Part model, mm, in its own coordinate system. A direction names the side the tool comes from. Give positions to 0.01 mm unless a question says otherwise; leave off trailing zeros. Write each loop counter-clockwise with the first axis right and the second up, starting at its lowest first coordinate (ties: lowest second). Pieces come first, ordered by that corner, then holes. Notation, with made-up numbers: (72, 87.25) - (109, 87.25) arc R29 cw to (109, 118.25) - close; hole circle Ø6 at (5, -9). An arc over 180 degrees is marked (long way). Answer in a Markdown table with one row per item. Add a question column.
1. Band-saw the part on C-C on z = 0.25. Write the cut outline in (x, y), plus the area to 3 significant figures.
2. Drop flat-ended pins along their axis: pin 1 Ø0.6 at (x, z) = (-1.5, -0.5) entering from -Y; pin 2 Ø1.7 at (x, z) = (0.5, 3) entering from -Y; pin 3 Ø1 at (x, z) = (4.5, 2.5) entering from -Y. Give the stop position or say it passes through.
3. Which spindle directions (+Z, -Z, +X, -X, +Y, -Y) get a long thin tool onto all of the face, cutting with end or side? Do faces 4 (the flat face through (-9.88, -1.16, 2.75)), 5 (the cylindrical face through (6.976, 2.754, 0.128)), 6 (the flat face through (-1, -10, -1.5)). Say none if no direction does.
4. Probe line 1 along X through (y, z) = (0, 2.75); line 2 along Z through (x, y) = (6.5, -4.25); line 3 along X through (y, z) = (4.5, -6). List the from-to ranges inside material, lowest first.
5. Band-saw the part on B-B on y = -8.5. Write the cut outline in (x, z), plus the area to 3 significant figures.
6. Pull direction Y, two halves, no side cores. Call faces 1 (the cylindrical face through (-0.857, -9.467, -0.021)), 2 (the cylindrical face through (7.614, -2.612, -1.705)), 3 (the flat face through (-1, -10, 1.5)): released by +Y, released by -Y, zero draft, split by the parting line, or undercut.
```python
from build123d import *

# Parameters (mm, degrees)
RESSALTO_EXTRUS_O1_DEPTH  = 10
CORTE_EXTRUS_O8_OUTLINE_W = 20
CORTE_EXTRUS_O8_OUTLINE_H = 20
CORTE_EXTRUS_O8_DEPTH     = 8.5
RESSALTO_EXTRUS_O2_START  = 1
RESSALTO_EXTRUS_O2_DEPTH  = 1
VARREDURA3_START          = -1.500007282
VARREDURA3_DEPTH          = 3
CORTE_EXTRUS_O9_DEPTH     = 15.5
FILETE1_R                 = 5


# Read off the part's stored shape, not the designer's step: Corte-extrusão8, Varredura3
with BuildPart() as part:
    # Esboço1 → Ressalto-extrusão1 (new, symmetric)
    with BuildSketch(Plane.XY):
        with BuildLine():
            Line((0, 8.5), (0, 7))
            Line((0, 7), (2.692582404, 7))
            ThreePointArc((2.692582404, 7), (7.373940602, -1.369306394), (0, -7.5))
            Line((0, -7.5), (0, -8.5))
            ThreePointArc((0, -8.5), (8.5, 0), (0, 8.5))
        make_face()
    extrude(amount=RESSALTO_EXTRUS_O1_DEPTH, both=True)

    # Corte-extrusão8 outline → Corte-extrusão8 (cut)
    with BuildSketch(Plane(origin=(0, 0, 0), x_dir=(0, 0, -1), z_dir=(1, 0, 0))):
        Rectangle(CORTE_EXTRUS_O8_OUTLINE_W, CORTE_EXTRUS_O8_OUTLINE_H)
        with BuildLine():
            add(Edge.make_bspline(
                [(9.000007282, 4.914510614), (9.447062759, 5.785868524), (9.685629081, 6.469892836)],
                knots=[0, 0, 0, 0.163868034, 0.163868034, 0.163868034], degree=2))
            add(Edge.make_bspline(
                [(3.935539792, -0.04688611), (4.779617707, 0.456269007), (6.467773537, 1.786323577), (8.155929367, 3.763866822), (9.000007282, 4.914510614)],
                knots=[0.718640695, 0.718640695, 0.718640695, 0.718640695, 0.859320348, 1, 1, 1, 1], degree=3))
            ThreePointArc((3.935539792, -0.04688611), (3.567999305, -0.305127766), (3.243137148, -0.615352428))
            Line((3.243137148, -0.615352428), (2.271512773, -1.693435261))
            ThreePointArc((2.271512773, -1.693435261), (1.699517724, -2.626111152), (1.500007282, -3.701870529))
            Line((1.500007282, -3.701870529), (-1.499992718, -3.701870529))
            ThreePointArc((-1.499992718, -3.701870529), (-1.69950316, -2.626111152), (-2.271498209, -1.693435261))
            Line((-2.271498209, -1.693435261), (-3.243122584, -0.615352428))
            ThreePointArc((-3.243122584, -0.615352428), (-3.567984742, -0.305127766), (-3.935525229, -0.04688611))
            add(Edge.make_bspline(
                [(-8.999992718, 4.914510614), (-8.155914803, 3.763866822), (-6.467758973, 1.786323577), (-4.779603143, 0.456269007), (-3.935525229, -0.04688611)],
                knots=[0, 0, 0, 0, 0.140679652, 0.281359305, 0.281359305, 0.281359305, 0.281359305], degree=3))
            add(Edge.make_bspline(
                [(-8.999992718, 4.914510614), (-9.619273552, 6.143045831), (-9.827290671, 7.002933405)],
                knots=[0, 0, 0, 0.226449118, 0.226449118, 0.226449118], degree=2))
            ThreePointArc((-9.827290671, 7.002933405), (-9.482547244, 8.038405471), (-8.484479959, 8.479894004))
            Line((-8.484479959, 8.479894004), (8.506836552, 8.482513232))
            ThreePointArc((8.506836552, 8.482513232), (9.673048984, 7.814043651), (9.685629081, 6.469892836))
        make_face(mode=Mode.SUBTRACT)
    extrude(amount=CORTE_EXTRUS_O8_DEPTH, mode=Mode.SUBTRACT)

    # Esboço22 → Ressalto-extrusão2 (add)
    with BuildSketch(Plane.ZY.offset(RESSALTO_EXTRUS_O2_START)):
        with BuildLine():
            Line((-9.85199593, 7), (9.826580108, 6.999999994))
            Line((9.826580108, 6.999999994), (9.827290671, 7.002933405))
            ThreePointArc((9.827290671, 7.002933405), (9.482547244, 8.038405471), (8.484479959, 8.479894004))
            Line((8.484479959, 8.479894004), (-8.506836552, 8.48251324))
            ThreePointArc((-8.506836552, 8.48251324), (-9.507748545, 8.039169154), (-9.85199593, 7))
        make_face()
    extrude(amount=-RESSALTO_EXTRUS_O2_DEPTH)

    # Espelhar17: part across plane


with BuildPart() as part_1:
    add(part.part)
    add(part.part.mirror(Plane(origin=(-1, 0, 0), x_dir=(0, 0, 1), z_dir=(1, 0, 0))))

    # Varredura3 outline → Varredura3 (add)
    with BuildSketch(Plane.XY.offset(VARREDURA3_START)):
        with BuildLine():
            ThreePointArc((6.52274134, -3.701870529), (6.829918041, -3.098744835), (7.081469689, -2.470381964))
            Line((7.081469689, -2.470381964), (6.760891253, -2.353494698))
            ThreePointArc((6.760891253, -2.353494698), (6.671498267, -3.032925038), (6.52274134, -3.701870529))
        make_face()
        with BuildLine():
            Line((7.651545895, -3.701870529), (6.52274134, -3.701870529))
            ThreePointArc((6.52274134, -3.701870529), (-1, -9.46822023), (-8.52274134, -3.701870529))
            Line((-8.52274134, -3.701870529), (-9.651545895, -3.701870529))
            ThreePointArc((-9.651545895, -3.701870529), (-1, -10.563106097), (7.651545895, -3.701870529))
        make_face()
    extrude(amount=VARREDURA3_DEPTH)

    # Esboço24 → Corte-extrusão9 (cut, symmetric)
    with BuildSketch(Plane.XY):
        with BuildLine():
            Line((-4.692582404, 7), (2.692582404, 7))
            ThreePointArc((2.692582404, 7), (4.307155609, 6.139903139), (5.665473098, 4.914510614))
            ThreePointArc((5.665473098, 4.914510614), (7.034580308, 2.600899823), (7.499853445, -0.04688611))
            ThreePointArc((7.499853445, -0.04688611), (7.492676559, -0.331357775), (7.474713465, -0.615352428))
            ThreePointArc((7.474713465, -0.615352428), (7.410147472, -1.157460341), (7.30631761, -1.693435261))
            ThreePointArc((7.30631761, -1.693435261), (6.987071698, -2.725954711), (6.52274134, -3.701870529))
            ThreePointArc((6.52274134, -3.701870529), (-1, -9.46822023), (-8.52274134, -3.701870529))
            ThreePointArc((-8.52274134, -3.701870529), (-8.987071698, -2.725954711), (-9.30631761, -1.693435261))
            ThreePointArc((-9.30631761, -1.693435261), (-9.410147472, -1.157460341), (-9.474713465, -0.615352428))
            ThreePointArc((-9.474713465, -0.615352428), (-9.492676559, -0.331357775), (-9.499853445, -0.04688611))
            ThreePointArc((-9.499853445, -0.04688611), (-9.034580308, 2.600899823), (-7.665473098, 4.914510614))
            ThreePointArc((-7.665473098, 4.914510614), (-6.307155609, 6.139903139), (-4.692582404, 7))
        make_face()
    extrude(amount=CORTE_EXTRUS_O9_DEPTH, both=True, mode=Mode.SUBTRACT)

    # Filete1
    filete1_edges = [part_1.edges().sort_by_distance(p)[0] for p in [
        (-4.692582404, 7, -0.01270694),
        (2.692582404, 7, -0.01270694),
    ]]
    fillet(filete1_edges, radius=FILETE1_R)


solid = part_1.part
```
Values:
| question | item | result |
|---|---|---|
| 1 | outline | (-9.65, -3.7) arc R8.89 ccw to (7.65, -3.7) arc R8.5 ccw to (0.57, 8.48) - (-2.57, 8.48) arc R8.5 ccw to start; hole (-8.52, -3.7) arc R7.79 ccw to (6.52, -3.7) arc R7.5 ccw to (4.5, 6) arc R5 ccw to (1.5, 7) - (-3.5, 7) arc R5 ccw to (-6.5, 6) arc R7.5 ccw to start |
| 1 | area | 62.1 mm² |
| 2 | pin 1 | stops at y = -10.56 |
| 2 | pin 2 | stops at y = 7 |
| 2 | pin 3 | stops at y = 5.59 |
| 3 | face 4 | +Z, +X, -X, -Y |
| 3 | face 5 | +Z, -Z |
| 3 | face 6 | -Z, +X, -X, -Y |
| 4 | line 1 | x = -10.5 to -9.5, 7.5 to 8.5 |
| 4 | line 2 | z = -1.5 to 1.5 |
| 4 | line 3 | x = -9.21 to -8, 6 to 7.21 |
| 5 | outline | (-6.69, -1.5) - (-4.76, -1.5) - (-4.76, 1.5) - (-6.69, 1.5) - close; (2.76, -1.5) - (4.69, -1.5) - (4.69, 1.5) - (2.76, 1.5) - close |
| 5 | area | 11.6 mm² |
| 6 | face 1 | undercut |
| 6 | face 2 | released by -Y |
| 6 | face 3 | zero draft |
